The model under review builds one solid part; all positions refer to its coordinate system, in mm. A direction names the side the tool comes from. Round coordinates to 2 decimals unless told otherwise and drop trailing zeros. Write each loop counter-clockwise with the first axis right and the second up, starting at its lowest first coordinate (ties: lowest second). Pieces come first, ordered by that corner, then holes. Notation, with made-up numbers: M 13.5,13.25 L 49.5,13.25 A23 ccw 49.5,29.25 Z; hole C 45,-22.75 d5. An arc over 180 degrees is marked long. Write item = value, one per line. Start each with the question number.
Item 1: Tool access review of faces 1 (the cylindrical face through (-40.519, 1.971, 6.194)), 2 (the cylindrical face through (-44.2, -7.2, 0)), 3 (the cylindrical face through (-44.2, 7.2, 0)), 4 (the flat face through (-63.8, -6, -3)): name each direction out of +Z, -Z, +X, -X, +Y, -Y from which nothing blocks a thin tool from reaching the whole face with its end or side.
Item 2: For pin 1 Ø3 at (y, z) = (0, 0) entering from +X; pin 2 Ø4 at (y, z) = (5.5, 0) entering from +X; pin 3 Ø4 at (y, z) = (-1.5, -1.5) entering from +X; pin 4 Ø1 at (y, z) = (1.5, 6) entering from +X, all flat-tipped, find the tip position at first contact; note any pin that passes through.
Item 3: Take a section at C-C, the plane y = 1.5. Give the boundary of the cut face in (x, z), plus the area to 3 significant figures.
Item 4: Take a section at A-A, the plane z = 0. Give the boundary of the cut face in (x, y).
Item 5: To check wall thickness, follow line 1 along X through (y, z) = (-4, -4.5); line 2 along Y through (x, z) = (-28, 4.25); line 3 along Z through (x, y) = (-40, -5). State the ranges of each line that lie inside material, in increasing order.
Item 6: The part is to be moulded in two halves that separate along Z. For faces 5 (the cylindrical face through (-44.2, 0, -7.2)), 6 (the flat face through (-24, -0.9, 6.6)), 7 (the flat face through (-62, 0, 3)), say which applies: +Z half, -Z half, draft (parallel to the pull), parting line (faces both ways), or undercut.
Item 7: Take a section at B-B, the plane x = -19. Give the boundary of the cut face in (y, z), plus the area to 3 significant figures.
Item 8: Take a section at D-D, the plane x = -59.5. Give the boundary of the cut face in (y, z).
Solid Edge part; units mm, degrees
sketch "Sketch1" plane through (0, 0, 0) normal (0, -1, 0) x (1, 0, 0)
  line L0 (-8, 7.6) -> (-63.8, 7.6)
  line L1 (-63.8, 7.6) -> (-63.8, 6.5)
  line L2 (-63.8, 6.5) -> (-64, 6.5)
  line L3 (-64, 2.4) -> (-64, 6.5)
  line L4 (-62, 2.4) -> (-64, 2.4)
  line L5 (-62, 6.5) -> (-62, 2.4)
  line L6 (-62, 6.5) -> (-24, 6.5)
  line L7 (-24, 6.5) -> (-14, 6.5)
  line L8 (-14, 6.5) -> (-14, 3.1)
  line L9 (-14, 3.1) -> (-8, 3.1)
  line L10 (0, 3.1) -> (-8, 3.1)
  line L11 (0, 3.1) -> (0, 6)
  line L12 (0, 6) -> (-8, 6)
  line L13 (-8, 6) -> (-8, 6.5)
  line L14 (-8, 6.5) -> (-8, 7.6)
revolve "RevolvedProtrusion1" add sketch "Sketch1" angle 360 about axis through (-64, 0, 0) along (1, 0, 0)
sketch "Sketch2" plane through (0, 0, 0) normal (0, 0, 1) x (1, 0, 0)
  line L0 (-16, 7.6) -> (-14, 14.7776)
  line L1 (-14, 14.7776) -> (20.3696, 14.7776)
  line L2 (20.3696, 14.7776) -> (20.3696, -22.0232)
  line L3 (20.3696, -22.0232) -> (-14, -21.4955)
  line L4 (-16, -7.6) -> (-14, -21.4955)
  line L5 (-24, -4) -> (-16, -7.6)
  line L6 (-24, 0) -> (-24, -4)
  line L7 (-24, 0) -> (-24, 4)
  line L8 (-24, 4) -> (-16, 7.6)
extrude "ExtrudedCutout_2" cut sketch "Sketch2" along normal mid plane 60
sketch "Sketch3" plane through (-24, 0, 6.3617) normal (1, 0, 0) x (0, 0, -1)
  line L0 (-0.7383, 0) -> (-0.7383, 0.4)
  line L1 (-0.7383, 0.4) -> (-0.1259, 0.4)
  line L2 (-0.7383, -0.4) -> (-0.1259, -0.4)
  line L3 (-0.7383, 0) -> (-0.7383, -0.4)
  arc A0 (-0.1259, 0.4) -> (-0.1259, -0.4) centre (6.3617, 0) ccw
extrude "ExtrudedCutout_3" add sketch "Sketch3" along normal blind 4
sketch "Sketch4" plane through (-20, 0, 6.3617) normal (1, 0, 0) x (0, 0, -1)
  line L0 (-0.7383, 0.4) -> (-1.2277, 0.4)
  line L1 (-0.7383, -0.4) -> (-1.2277, -0.4)
  line L2 (-0.7383, 0.4) -> (-0.7383, -0.4)
  arc A0 (-1.2277, 0.4) -> (-1.2277, -0.4) centre (6.3617, 0) ccw
extrude "ExtrudedProtrusion_3" add sketch "Sketch4" against normal blind 0.8
mirror "Mirror1" about plane through (0, 0, 0) normal (0, 0, 1) of "ExtrudedProtrusion_3", "ExtrudedCutout_3"
sketch "Sketch5" plane through (-64, 0, 0) normal (-1, 0, 0) x (0, -1, 0)
  line L0 (6.7658, 2.4625) -> (7.1417, 2.5994)
  arc A0 (7.1417, 2.5994) -> (7.1417, -2.5994) centre (0, 0) cw
  line L1 (6.7658, -2.4625) -> (7.1417, -2.5994)
  arc A1 (6.7658, 2.4625) -> (6.7658, -2.4625) centre (0, 0) cw
  line L2 (2.4625, -6.7658) -> (2.5994, -7.1417)
  arc A2 (2.5994, -7.1417) -> (-2.5994, -7.1417) centre (0, 0) cw
  line L3 (-2.4625, -6.7658) -> (-2.5994, -7.1417)
  arc A3 (2.4625, -6.7658) -> (-2.4625, -6.7658) centre (0, 0) cw
  line L4 (-6.7658, -2.4625) -> (-7.1417, -2.5994)
  line L5 (-6.7658, 2.4625) -> (-7.1417, 2.5994)
  arc A4 (-6.7658, 2.4625) -> (-6.7658, -2.4625) centre (0, 0) ccw
  arc A5 (-7.1417, -2.5994) -> (-7.1417, 2.5994) centre (0, 0) cw
  line L6 (-2.4625, 6.7658) -> (-2.5994, 7.1417)
  arc A6 (-2.5994, 7.1417) -> (2.5994, 7.1417) centre (0, 0) cw
  line L7 (2.4625, 6.7658) -> (2.5994, 7.1417)
  arc A7 (-2.4625, 6.7658) -> (2.4625, 6.7658) centre (0, 0) cw
extrude "ExtrudedCutout_4" cut sketch "Sketch5" against normal blind 40
Response values:
q1.face_1 = +X
q1.face_2 = -X, -Y
q1.face_3 = -X, +Y
q1.face_4 = -X
q2.pin_1 = through
q2.pin_2 = -16.22
q2.pin_3 = -62
q2.pin_4 = -24
q3.outline = M -64,-6.32 L -63.8,-6.32 L -63.8,-7.04 L -24,-7.04 L -24,-6.32 L -62,-6.32 L -62,-1.87 L -64,-1.87 Z; M -64,1.87 L -62,1.87 L -62,6.32 L -24,6.32 L -24,7.04 L -63.8,7.04 L -63.8,6.32 L -64,6.32 Z
q3.area = 74.9 mm2
q4.outline = M -64,-6.5 L -63.8,-6.5 L -63.8,-7.2 L -24,-7.2 L -24,-7.6 L -16,-7.6 L -18.44,-6.5 L -62,-6.5 L -62,-2.4 L -64,-2.4 Z; M -64,2.4 L -62,2.4 L -62,6.5 L -18.44,6.5 L -16,7.6 L -24,7.6 L -24,7.2 L -63.8,7.2 L -63.8,6.5 L -64,6.5 Z
q5.line_1 = -64 to -62
q5.line_2 = -6.3 to -4.92, 4.92 to 6.3
q5.line_3 = -5.72 to -4.15, 4.15 to 5.72
q6.face_5 = -Z half
q6.face_6 = draft
q6.face_7 = undercut
q7.outline = M -6.25,-4.32 L -6.25,-1.79 A6.5 cw -6.25,1.79 L -6.25,4.32 A7.6 ccw Z; M 6.25,-4.32 A7.6 ccw 6.25,4.32 L 6.25,1.79 A6.5 cw 6.25,-1.79 Z
q7.area = 14.7 mm2
q8.outline = M -7.14,-2.6 A7.6 ccw -2.6,-7.14 L -2.46,-6.77 A7.2 ccw 2.46,-6.77 L 2.6,-7.14 A7.6 ccw 7.14,-2.6 L 6.77,-2.46 A7.2 ccw 6.77,2.46 L 7.14,2.6 A7.6 ccw 2.6,7.14 L 2.46,6.77 A7.2 ccw -2.46,6.77 L -2.6,7.14 A7.6 ccw -7.14,2.6 L -6.77,2.46 A7.2 ccw -6.77,-2.46 Z; hole C 0,0 d13
